```python
from build123d import *

# Parameters (mm, degrees)
ESQUISSE2_R             = 18.25
BOSS_EXTRU_1_DEPTH      = 5.25
ESQUISSE3_R             = 17.25
BOSS_EXTRU_2_DEPTH      = 9
ESQUISSE4_R             = 18.25
BOSS_EXTRU_3_DEPTH      = 5.25
ESQUISSE6_R             = 1.5
BOSS_EXTRU_4_DEPTH      = 2
ESQUISSE7_R             = 8
BOSS_EXTRU_5_DEPTH      = 2
ESQUISSE8_R             = 2.5
BOSS_EXTRU_6_DEPTH      = 15
CHANFREIN1_SIZE         = 0.25
ESQUISSE9_W             = 5
ESQUISSE9_H             = 1
ENL_V_MAT_EXTRU_1_DEPTH = 10


with BuildPart() as part:
    # Esquisse2 → Boss.-Extru.1 (new body)
    with BuildSketch(Plane(origin=(0, 0, 0), x_dir=(0, 0, -1), z_dir=(1, 0, 0))):
        with Locations(Location((0, 0, 0), (0, 0, 180))):
            Circle(ESQUISSE2_R)
    extrude(amount=BOSS_EXTRU_1_DEPTH)

    # Esquisse3 → Boss.-Extru.2 (add)
    with BuildSketch(Plane(origin=(5.25, 0, 0), x_dir=(0, 0, -1), z_dir=(1, 0, 0))):
        Circle(ESQUISSE3_R)
    extrude(amount=BOSS_EXTRU_2_DEPTH)

    # Esquisse4 → Boss.-Extru.3 (add)
    with BuildSketch(Plane(origin=(14.25, 0, 0), x_dir=(0, 0, -1), z_dir=(1, 0, 0))):
        with Locations(Location((0, 0, 0), (0, 0, 180))):
            Circle(ESQUISSE4_R)
    extrude(amount=BOSS_EXTRU_3_DEPTH)

    # Esquisse6 → Boss.-Extru.4 (add)
    # profile 1 of 2: a face of its own
    with BuildSketch(Plane.ZY):
        with BuildLine():
            ThreePointArc((23.313667029, -3.27763821), (25.5, 0), (23.313667029, 3.27763821))
            Line((23.313667029, 3.27763821), (17.312357631, 5.774493333))
            ThreePointArc((17.312357631, 5.774493333), (18.014064322, 2.925061814), (18.25, 0))
            ThreePointArc((18.25, 0), (18.014064322, -2.925061814), (17.312357631, -5.774493333))
            Line((17.312357631, -5.774493333), (23.313667029, -3.27763821))
        make_face()
        with Locations((21.95, 0)):
            Circle(ESQUISSE6_R, mode=Mode.SUBTRACT)
    # profile 2 of 2: a face of its own
    with BuildSketch(Plane.ZY):
        with BuildLine():
            ThreePointArc((-17.312357631, -5.774493333), (-18.25, 0), (-17.312357631, 5.774493333))
            Line((-17.312357631, 5.774493333), (-23.313667029, 3.27763821))
            ThreePointArc((-23.313667029, 3.27763821), (-25.5, 0), (-23.313667029, -3.27763821))
            Line((-23.313667029, -3.27763821), (-17.312357631, -5.774493333))
        make_face()
        with Locations((-21.95, 0)):
            Circle(ESQUISSE6_R, mode=Mode.SUBTRACT)
    extrude(amount=-BOSS_EXTRU_4_DEPTH)

    # Esquisse7 → Boss.-Extru.5 (add)
    with BuildSketch(Plane.ZY):
        Circle(ESQUISSE7_R)
    extrude(amount=BOSS_EXTRU_5_DEPTH)

    # Esquisse8 → Boss.-Extru.6 (add)
    with BuildSketch(Plane.ZY):
        Circle(ESQUISSE8_R)
    extrude(amount=BOSS_EXTRU_6_DEPTH)

    # Chanfrein1
    chanfrein1_edges = [part.edges().sort_by_distance(p)[0] for p in [
        (-15, 0, -2.5),
    ]]
    chamfer(chanfrein1_edges, length=CHANFREIN1_SIZE)

    # Esquisse9 → Enlèv. mat.-Extru.1 (cut)
    with BuildSketch(Plane.ZY.offset(15)):
        with Locations((0, 2.5)):
            Rectangle(ESQUISSE9_W, ESQUISSE9_H)
    extrude(amount=-ENL_V_MAT_EXTRU_1_DEPTH, mode=Mode.SUBTRACT)


solid = part.part
```
CAD build for the part. Positions are in the model's coordinates, mm. A direction names the side the tool comes from. Round coordinates to 2 decimals unless told otherwise and drop trailing zeros. Order: outer loops, then holes, each group sorted by start corner. A loop starts at its lowest first (then second) coordinate and runs counter-clockwise, first axis right, second up.
Item 1: Saw through at A-A on z = 22. Write the cut outline in (x, y), then the cut area to 3 significant figures.
Item 2: Saw through at C-C on z = 0. Write the cut outline in (x, y).
Item 3: Tool access for faces 5 (the face through (1, -0.1, 25.5)), 6 (the face through (9.687, 5.181, -16.453)), 7 (the face through (-10, 2, 0)), 8 (the face through (2.6, 16.2, 8.4)), 9 (the face through (-2, 2, 2)): list every direction of +Z, -Z, +X, -X, +Y, -Y with a clear straight run to the whole face (end or side of a thin tool).
Item 4: Saw through at B-B on y = -12. Write the cut outline in (x, z), then the cut area to 3 significant figures.
Item 5: Pin check, flat tips, straight feed: pin 1 (3 mm diameter, centred on y = 13.5, z = -10.5, fed in from -X); pin 2 (3 mm diameter, centred on x = 0, z = 9, fed in from +Y); pin 3 (0.9 mm diameter, centred on x = -10.5, z = 0.5, fed in from +Y); pin 4 (1.8 mm diameter, centred on y = 0, z = -21.95, fed in from +X). Stop position of each tip, or through.
Item 6: Probe line 1 along X through (y, z) = (1, -17.5); line 2 along X through (y, z) = (-9.5, 4.5); line 3 along Y through (x, z) = (1.5, 21.95) (3 decimals). List the from-to ranges inside material, lowest first.
Item 7: Saw through at D-D on x = -9.5. Write the cut outline in (y, z).
Item 8: Mould opens along Y. For faces 1 (the face through (-0.99, -7.81, -1.73)), 2 (the face through (0.99, 0.45, -20.52)), 3 (the face through (19.5, 0, 0)), 4 (the face through (0.99, 0.07, 20.45)) say: pulls with the +Y half, pulls with the -Y half, needs draft (parallel to the pull), parting line crosses it, or undercut.
Reported:
1. outline: (0, -3.82) - (2, -3.82) - (2, -1.5) - (0, -1.5) - close; (0, 1.5) - (2, 1.5) - (2, 3.82) - (0, 3.82) - close
1. area: 9.30 mm2
2. outline: (-15, -2.25) - (-14.75, -2.5) - (-2, -2.5) - (-2, -8) - (0, -8) - (0, -18.25) - (5.25, -18.25) - (5.25, -17.25) - (14.25, -17.25) - (14.25, -18.25) - (19.5, -18.25) - (19.5, 18.25) - (14.25, 18.25) - (14.25, 17.25) - (5.25, 17.25) - (5.25, 18.25) - (0, 18.25) - (0, 8) - (-2, 8) - (-2, 2.5) - (-5, 2.5) - (-5, 2) - (-15, 2) - close
3. face 5: +Z, +X, -X
3. face 6: none
3. face 7: +Z, -Z, -X, +Y
3. face 8: +X
3. face 9: -X
4. outline: (0, -13.75) - (5.25, -13.75) - (5.25, -12.39) - (14.25, -12.39) - (14.25, -13.75) - (19.5, -13.75) - (19.5, 13.75) - (14.25, 13.75) - (14.25, 12.39) - (5.25, 12.39) - (5.25, 13.75) - (0, 13.75) - close
4. area: 512 mm2
5. pin 1: stops at x = 0
5. pin 2: stops at y = 16.64
5. pin 3: stops at y = 2
5. pin 4: passes through
6. line 1: x = 0 to 5.25, 14.25 to 19.5
6. line 2: x = 0 to 19.5
6. line 3: y = -3.845 to -1.5, 1.5 to 3.845
7. outline: (2, -1.5) - (2, 1.5) arc R2.5 ccw (long way) to start
8. face 1: parting line crosses it
8. face 2: undercut
8. face 3: needs draft
8. face 4: undercut
